Solid Edge part; units mm, degrees
sketch "Sketch1" plane through (0, 0, 0) normal (0, 0, 1) x (1, 0, 0)
  line L0 (-17.5, 29.75) -> (17.5, 29.75)
  line L1 (17.5, 29.75) -> (17.5, 14.75)
  line L2 (17.5, 14.75) -> (22.3, 14.75)
  line L3 (22.3, -0.25) -> (22.3, 14.75)
  line L4 (22.3, -0.25) -> (22.3, -15.25)
  line L5 (22.3, -15.25) -> (17.5, -15.25)
  line L6 (17.5, -30.25) -> (17.5, -15.25)
  line L7 (-17.5, -30.25) -> (17.5, -30.25)
  line L8 (-17.5, -15.25) -> (-17.5, -30.25)
  line L9 (-22.3, -15.25) -> (-17.5, -15.25)
  line L10 (-22.3, -0.25) -> (-22.3, -15.25)
  line L11 (-22.3, -0.25) -> (-22.3, 14.75)
  line L12 (-17.5, 14.75) -> (-22.3, 14.75)
  line L13 (-17.5, 14.75) -> (-17.5, 29.75)
  circle A0 centre (3.45, 14.16) radius 1.25
  circle A1 centre (-7.895, 10.74) radius 1.25
  circle A2 centre (-3.45, -14.66) radius 1.25
  circle A3 centre (7.895, -11.24) radius 1.25
extrude "ExtrudedProtrusion_6" add sketch "Sketch1" along normal blind 4.8
sketch "Sketch2" plane through (0, 0, 4.8) normal (0, 0, 1) x (1, 0, 0)
  line L0 (-19.9, 14.75) -> (-19.9, -15.25)
  line L1 (-19.9, -15.25) -> (-17.5, -15.25)
  line L2 (-17.5, -15.25) -> (-17.5, 14.75)
  line L3 (-17.5, 14.75) -> (-19.9, 14.75)
  line L4 (19.9, -15.25) -> (19.9, 14.75)
  line L5 (19.9, 14.75) -> (17.5, 14.75)
  line L6 (17.5, 14.75) -> (17.5, -15.25)
  line L7 (17.5, -15.25) -> (19.9, -15.25)
extrude "ExtrudedCutout_5" cut sketch "Sketch2" against normal blind 2.4
sketch "Sketch3" plane through (0, -0.25, 4.8) normal (0, 0, 1) x (1, 0, 0)
  line L0 (6.4059, 8.4485) -> (-9.8703, 3.5406)
  arc A0 (-13.2139, -2.69) -> (-9.8703, 3.5406) centre (-8.4268, -1.2465) cw
  line L1 (-13.2139, -2.69) -> (-12.6365, -4.6048)
  arc A1 (-12.6365, -4.6048) -> (-6.4059, -7.9485) centre (-7.8494, -3.1614) ccw
  line L2 (-6.4059, -7.9485) -> (9.8703, -3.0406)
  arc A2 (9.8703, -3.0406) -> (13.2139, 3.19) centre (8.4268, 1.7465) ccw
  line L3 (13.2139, 3.19) -> (12.6365, 5.1048)
  arc A3 (6.4059, 8.4485) -> (12.6365, 5.1048) centre (7.8494, 3.6614) cw
extrude "ExtrudedCutout_7" cut sketch "Sketch3" against normal blind 5
sketch "Sketch4" plane through (0, -30.25, 2.4) normal (0, -1, 0) x (-1, 0, 0)
  circle A0 centre (0, 0) radius 1.25
extrude "ExtrudedCutout_8" cut sketch "Sketch4" against normal blind 12
properties material "Polycarbonate"
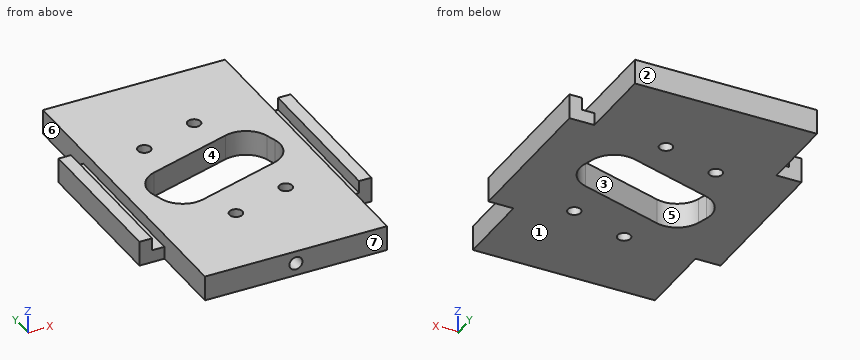
Work out the finished part from the listing and answer in its coordinate system (mm). Face numbers are marked on the shaded views. A direction names the side the tool comes from. Coordinates: 2 decimals unless noted, no trailing zeros. Loops run counter-clockwise (first coordinate to the right, second up) from the corner with the lowest first, then second, coordinate; pieces in that order, holes last. Notation, with made-up numbers: M -8.5,56 L 36.5,56 A26 ccw 36.5,94 Z; hole C -27.75,-18.5 d7. An arc over 180 degrees is marked long. Answer in a Markdown table with one row per item. Add a question column.
1. Flat-ended cylindrical pins translate along their axes: P1, Ø2, axis at x = -3.45, y = -14.66, coming from the -Z side; P2, Ø2.5, axis at x = 20.5, z = 2.5, coming from the +Y side. Find the tip coordinate at first contact, or state that the pin passes through.
2. Consider L1, parallel to Y at x = 3.5, z = 0.75; L2, parallel to Y at x = -3.45, z = 2.7; L3, parallel to Y at x = 20.5, z = 2.1. Determine where each line is inside the solid, lowest interval first.
3. Find section B-B, the plane x = 0. Write down the section's boundary in (y, z).
4. The mould has two halves that part along Y. Classify the marked faces 1, 2, 3 and 4: pulls with the +Y half, pulls with the -Y half, needs draft (parallel to the pull), parting line crosses it, or undercut.
5. Find section C-C, the plane y = -26. Write down the section's boundary in (x, z).
6. A tool of negligible diameter and unlimited length cuts with its end or side. For the marked faces 5, 6 and 7, from which of +Z, -Z, +X, -X, +Y, -Y can it reach the whole face along a straight path? Write none if from no direction.
7. Find section D-D, the plane y = -2. Write down the section's boundary in (x, z), then the cut area to 3 significant figures.
8. Find section A-A, the plane y = 10.74. Write down the section's boundary in (x, z) (3 decimals), then the cut area to 3 significant figures.
Reported:
| question | item | result |
|---|---|---|
| 1 | P1 | passes through |
| 1 | P2 | stops at y = 14.75 |
| 2 | L1 | y = -30.25 to -5.21, 7.32 to 12.91, 15.41 to 29.75 |
| 2 | L2 | y = -30.25 to -15.91, -13.41 to -7.31, 5.23 to 29.75 |
| 2 | L3 | y = -15.25 to 14.75 |
| 3 | outline | M -30.25,0 L -6.27,0 L -6.27,4.8 L -30.25,4.8 L -30.25,3.65 L -18.25,3.65 L -18.25,1.15 L -30.25,1.15 Z; M 6.27,0 L 29.75,0 L 29.75,4.8 L 6.27,4.8 Z |
| 4 | face 1 | needs draft |
| 4 | face 2 | pulls with the +Y half |
| 4 | face 3 | undercut |
| 4 | face 4 | undercut |
| 5 | outline | M -17.5,0 L 17.5,0 L 17.5,4.8 L -17.5,4.8 Z; hole C 0,2.4 d2.5 |
| 6 | face 5 | +Z, -Z |
| 6 | face 6 | +Z |
| 6 | face 7 | +Z, -Z, +X, -X, -Y |
| 7 | outline | M -22.3,0 L -13.4,0 L -13.4,4.8 L -17.5,4.8 L -17.5,2.4 L -19.9,2.4 L -19.9,4.8 L -22.3,4.8 Z; M 12,0 L 22.3,0 L 22.3,4.8 L 19.9,4.8 L 19.9,2.4 L 17.5,2.4 L 17.5,4.8 L 12,4.8 Z |
| 7 | area | 80.6 mm^2 |
| 8 | outline | M -22.3,0 L -9.145,0 L -9.145,4.8 L -17.5,4.8 L -17.5,2.4 L -19.9,2.4 L -19.9,4.8 L -22.3,4.8 Z; M -6.645,0 L 22.3,0 L 22.3,4.8 L 19.9,4.8 L 19.9,2.4 L 17.5,2.4 L 17.5,4.8 L -6.645,4.8 Z |
| 8 | area | 191 mm^2 |
